Here's how the part is built. I have some questions about the finished solid (model axes, mm). A direction names the side the tool comes from. Round coordinates to 2 decimals unless told otherwise and drop trailing zeros. Order: outer loops, then holes, each group sorted by start corner. A loop starts at its lowest first (then second) coordinate and runs counter-clockwise, first axis right, second up. Notation, with made-up numbers: M -13.75,22.5 L 20.25,22.5 A17 cw 20.25,48.5 Z; hole C 17,-26.5 d3. An arc over 180 degrees is marked long. Use one line per item in the form item = value. Start each with the question number.
```python
from build123d import *

# Parameters (mm, degrees)
SKETCH2_R           = 2.1
BOSS_EXTRUDE1_DEPTH = 26
SKETCH3_W           = 7.4
SKETCH3_H           = 18
SKETCH3_W_2         = 7.8
SKETCH3_W_3         = 7.481047655
CUT_EXTRUDE1_DEPTH  = 17
SKETCH4_W           = 26
SKETCH4_H           = 9
BOSS_EXTRUDE2_DEPTH = 25
SKETCH5_W           = 19
SKETCH5_H           = 6
CUT_EXTRUDE2_DEPTH  = 25
FILLET1_R           = 3
FILLET2_R           = 3
FILLET3_R           = 0.5
SKETCH6_R           = 1.5
CUT_EXTRUDE3_DEPTH  = 12.5


with BuildPart() as part:
    # Sketch2 → Boss-Extrude1 (new body, symmetric)
    with BuildSketch(Plane(origin=(0, 0, 0), x_dir=(0, 0, -1), z_dir=(1, 0, 0))):
        with BuildLine():
            Line((-8, 0), (-8, 20))
            Line((-8, 20), (8, 20))
            Line((8, 20), (8, 0))
            ThreePointArc((8, 0), (0, -8), (-8, 0))
        make_face()
        Circle(SKETCH2_R, mode=Mode.SUBTRACT)
    extrude(amount=BOSS_EXTRUDE1_DEPTH, both=True)

    # Sketch3 → Cut-Extrude1 (cut, through all)
    with BuildSketch(Plane.XY.offset(8)):
        with Locations((-22.3, 0)):
            Rectangle(SKETCH3_W, SKETCH3_H)
        with Locations((-7.5, 0)):
            Rectangle(SKETCH3_W_2, SKETCH3_H)
        with Locations((7.5, 0)):
            Rectangle(SKETCH3_W_2, SKETCH3_H)
        with Locations((22.259476173, 0)):
            Rectangle(SKETCH3_W_3, SKETCH3_H)
    extrude(amount=-CUT_EXTRUDE1_DEPTH, mode=Mode.SUBTRACT)

    # Sketch4 → Boss-Extrude2 (add)
    with BuildSketch(Plane(origin=(0, 20, 0), x_dir=(1, 0, 0), z_dir=(0, 1, 0))):
        with Locations((0, -3.5)):
            Rectangle(SKETCH4_W, SKETCH4_H)
    extrude(amount=BOSS_EXTRUDE2_DEPTH)

    # Sketch5 → Cut-Extrude2 (cut)
    with BuildSketch(Plane(origin=(0, 45, 0), x_dir=(1, 0, 0), z_dir=(0, 1, 0))):
        with Locations((0, -5)):
            Rectangle(SKETCH5_W, SKETCH5_H)
    extrude(amount=-CUT_EXTRUDE2_DEPTH, mode=Mode.SUBTRACT)

    # Fillet1
    fillet1_edges = [part.edges().sort_by_distance(p)[0] for p in [
        (-13, 20, 3.5),
        (13, 20, 3.5),
        (0, 20, -1),
    ]]
    fillet(fillet1_edges, radius=FILLET1_R)

    # Fillet2
    fillet2_edges = [part.edges().sort_by_distance(p)[0] for p in [
        (26, 20, 0),
        (-26, 20, 0),
    ]]
    fillet(fillet2_edges, radius=FILLET2_R)

    # Fillet3
    fillet3_edges = [part.edges().sort_by_distance(p)[0] for p in [
        (-13, 45, 3.5),
        (-11.25, 45, 8),
        (13, 45, 3.5),
        (0, 45, -1),
        (11.25, 45, 8),
        (9.5, 45, 5),
        (0, 45, 2),
        (-9.5, 45, 5),
    ]]
    fillet(fillet3_edges, radius=FILLET3_R)

    # Sketch6 → Cut-Extrude3 (cut, symmetric)
    with BuildSketch(Plane.XY):
        with Locations((0, 37.5)):
            Circle(SKETCH6_R)
        with Locations((0, 27.5)):
            Circle(SKETCH6_R)
    extrude(amount=CUT_EXTRUDE3_DEPTH, both=True, mode=Mode.SUBTRACT)


solid = part.part
```
1) On a 3-axis mill with a long thin cutter (end or side, diameter ignored), from which of +Z, -Z, +X, -X, +Y, -Y can I reach the whole of each face in a straight line? I mean faces 1 (the flat face through (22, 9, 0)), 2 (the flat face through (9.5, 32, 5)), 3 (the flat face through (0, 34, -1)), 4 (the flat face through (3.6, 2.3, 0.1)). Say none if no direction works.
2) If we section it at C-C on y = 24: Write out the boundary of the cut face in (x, z), then the cut area to 3 significant figures.
3) If we section it at D-D on x = 17.5: Write out the boundary of the cut face in (y, z).
4) If I drill on line 1 (X direction, y = 6.5, z = 4); line 2 (Y direction, x = -16.25, z = 0); line 3 (Y direction, x = 0, z = 0.6), over which ranges is the centre line in solid material (lowest first)?
5) If we section it at A-A on y = 37.5: Write out the boundary of the cut face in (x, z).
6) If we section it at B-B on x = 0: Write out the boundary of the cut face in (y, z).
7) Will these pins go through, and if not, where does the flat tip stop? pin 1 Ø2 at (x, z) = (-23, 3.5) entering from -Y; pin 2 Ø7 at (y, z) = (37.5, 4.5) entering from +X; pin 3 Ø5 at (y, z) = (2, -1) entering from -X; pin 4 Ø3.5 at (y, z) = (0, 0) entering from -X.
8) If we mould it in two halves opening along Z, with no side actions, what happens to faces 5 (the cylindrical face through (0, 36, 1)), 6 (the cylindrical face through (-15.05, 0.631, -2.003)), 7 (the cylindrical face through (0.22, 20.86, -1.9))? For each: +Z half, -Z half, draft (parallel to the pull), parting line (faces both ways), or undercut.
Completed:
q1.face_1 = +Z, -Z, +X, -Y
q1.face_2 = +Z, +Y
q1.face_3 = -Z, +X, -X, +Y
q1.face_4 = +Z, -Z, -Y
q2.outline = M -13,-1 L 13,-1 L 13,8 L 9.5,8 L 9.5,2 L -9.5,2 L -9.5,8 L -13,8 Z
q2.area = 120 mm²
q3.outline = M 0,-8 L 20,-8 L 20,8 L 0,8 A8 ccw Z; hole C 0,0 d4.2
q4.line_1 = -18.6 to -11.4, -3.6 to 3.6, 11.4 to 18.52
q4.line_2 = -8 to -2.1, 2.1 to 20
q4.line_3 = -7.98 to -2.01, 2.01 to 26, 29 to 36, 39 to 45
q5.outline = M -13,-1 L -1.5,-1 L -1.5,2 L -9.5,2 L -9.5,8 L -13,8 Z; M 1.5,-1 L 13,-1 L 13,8 L 9.5,8 L 9.5,2 L 1.5,2 Z
q6.outline = M 0,-8 L 20,-8 L 20,-4 A3 cw 23,-1 L 26,-1 L 26,2 L 20,2 L 20,8 L 0,8 A8 ccw Z; M 29,-1 L 36,-1 L 36,2 L 29,2 Z; M 39,-1 L 44.5,-1 A0.5 ccw 45,-0.5 L 45,1.5 A0.5 ccw 44.5,2 L 39,2 Z; hole C 0,0 d4.2
q7.pin_1 = 9
q7.pin_2 = 13
q7.pin_3 = -18.6
q7.pin_4 = through
q8.face_5 = draft
q8.face_6 = undercut
q8.face_7 = -Z half
